from build123d import *

# Parameters (mm, degrees)
F0_R     = 15
F1_DEPTH = 4
F2_R     = 3
F3_DEPTH = 1.5
F4_T     = -1
F5_DEPTH = 1.5


with BuildPart() as f1:
    # F0 (on Top) → F1 (new body)
    with BuildSketch(Plane.XY):
        Circle(F0_R)
    extrude(amount=F1_DEPTH)

    # F2
    f2_edges = [f1.edges().sort_by_distance(p)[0] for p in [
        (-15, 0, 4),
    ]]
    fillet(f2_edges, radius=F2_R)

    # F3 (cut): a face of the model
    f3_faces = [f1.faces().sort_by_distance(p)[0] for p in [
        (0, 0, 4),
    ]]
    extrude(f3_faces, amount=-F3_DEPTH, mode=Mode.SUBTRACT)

    # F4
    f4_openings = [f1.faces().sort_by_distance(p)[0] for p in [
        (0, 0, 0),
    ]]
    offset(amount=F4_T, openings=f4_openings, kind=Kind.INTERSECTION)

    # F5 (add): a face of the model
    f5_faces = [f1.faces().sort_by_distance(p)[0] for p in [
        (0, 0, 1.5),
    ]]
    extrude(f5_faces, amount=F5_DEPTH)


solid = f1.part
Geometry check sheet. Reference: the model listing, model coordinates, mm. A direction names the side the tool comes from. Give positions to 0.01 mm unless a question says otherwise; leave off trailing zeros. Loops run counter-clockwise (first coordinate to the right, second up) from the corner with the lowest first, then second, coordinate; pieces in that order, holes last. Notation, with made-up numbers: (-3.75, -36.5) -> (54.25, -36.5) arc R14 ccw to (54.25, -17.5) -> close; hole circle Ø3 at (73.25, -28). An arc over 180 degrees is marked (long way). Answer in a Markdown table with one row per item. Add a question column.
1) Gauge pin test, flat ends, axial feed: P1, Ø2, axis at x = -1, z = 2.5, coming from the -Y side; P2, Ø2, axis at x = 7, y = -5.5, coming from the -Z side; P3, Ø3, axis at x = 4.5, y = -3.5, coming from the +Z side; P4, Ø1.5, axis at y = 5, z = 2, coming from the -X side. Record the tip position at first contact, or that the pin passes through.
2) Cross-section at D-D on z = 3.1. Record the boundary of the cut face in (x, y).
3) Set-up check for faces 4 (the face through (-11.99, 0.53, 3.26)), 5 (the face through (-10.316, -7.91, 1.385)): record each of +Z, -Z, +X, -X, +Y, -Y from which the full face is reachable in a straight line by a thin tool's end or side.
4) Cross-section at B-B on x = 0. Record the boundary of the cut face in (y, z).
5) Material ranges on probe 1 along Y at (x, z) = (0, 0.7); probe 2 along X at (y, z) = (3.75, 1.35); probe 3 along Y at (x, z) = (8, 2.65), recorded low to high. Write a range as from..to.
6) Draft check along X on faces 1 (the face through (0, 0, 0)), 2 (the face through (12.932, -5.362, 0.493)), 3 (the face through (-14.985, 0.66, 0.493)). Enter one of: pulls with the +X half, pulls with the -X half, needs draft (parallel to the pull), parting line crosses it, or undercut.
7) Cross-section at A-A on z = 0.45. Record the boundary of the cut face in (x, y), and give its area (3 significant figures).
Outcome:
| question | item | result |
|---|---|---|
| 1 | P1 | stops at y = -14.93 |
| 1 | P2 | stops at z = 0 |
| 1 | P3 | stops at z = 2.5 |
| 1 | P4 | stops at x = -14.29 |
| 2 | outline | circle Ø28.28 at (0, 0); hole circle Ø24 at (0, 0) |
| 3 | face 4 | +Z |
| 3 | face 5 | -Z |
| 4 | outline | (-15, 0) -> (-14, 0) -> (-14, 1) arc R2 cw to (-13, 2.73) -> (-13, 0) -> (13, 0) -> (13, 2.73) arc R2 cw to (14, 1) -> (14, 0) -> (15, 0) -> (15, 1) arc R3 ccw to (12, 4) -> (12, 2.5) -> (-12, 2.5) -> (-12, 4) arc R3 ccw to (-15, 1) -> close |
| 5 | probe 1 | y = -15..-14, -13..13, 14..15 |
| 5 | probe 2 | x = -14.5..-13.46, -12.45..12.45, 13.46..14.5 |
| 5 | probe 3 | y = -12.1..-10.41, -10.25..-8.94, 8.94..10.25, 10.41..12.1 |
| 6 | face 1 | needs draft |
| 6 | face 2 | undercut |
| 6 | face 3 | parting line crosses it |
| 7 | outline | circle Ø30 at (0, 0); circle Ø26 at (0, 0); hole circle Ø28 at (0, 0) |
| 7 | area | 622 mm^2 |
